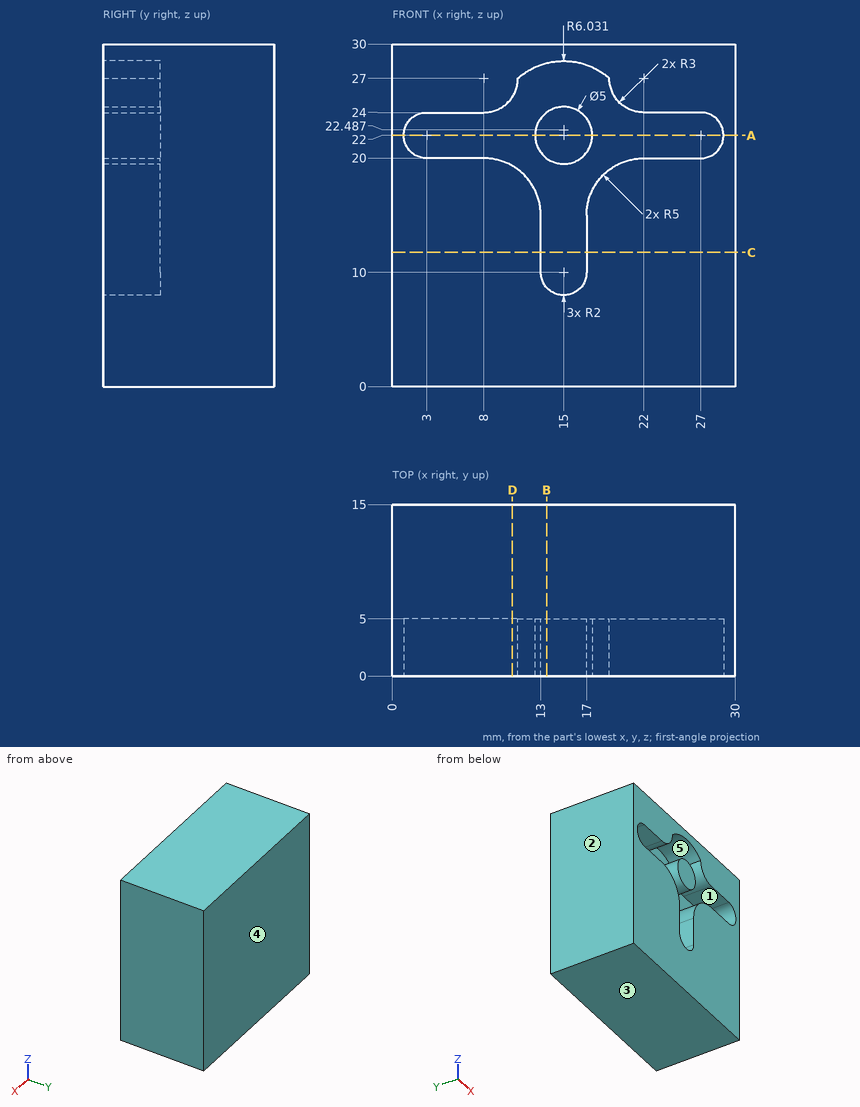
Here's the drawing with two shaded views (mm, measured from the low corner). I have some questions. A direction names the side the tool comes from. Coordinates: 2 decimals unless noted, no trailing zeros. Write each loop counter-clockwise with the first axis right and the second up, starting at its lowest first coordinate (ties: lowest second). Pieces come first, ordered by that corner, then holes.
Item 1: I want a section at C-C on z = 11.75. Write out the boundary of the cut face in (x, y), and give its area (3 significant figures).
Item 2: I want a section at B-B on x = 13.5. Write out the boundary of the cut face in (y, z).
Item 3: If I drill on line 1 (X direction, y = 4.5, z = 14.5); line 2 (Z direction, x = 26.5, y = 0.5); line 3 (Y direction, x = 21.75, z = 23.5), over which ranges is the centre line in solid material (lowest first)?
Item 4: If we mould it in two halves opening along Z, with no side actions, what happens to the marked faces 1, 2 and 3? For each: +Z half, -Z half, draft (parallel to the pull), parting line (faces both ways), or undercut.
Item 5: I want a section at D-D on x = 10.5. Write out the boundary of the cut face in (y, z).
Item 6: On a 3-axis mill with a long thin cutter (end or side, diameter ignored), from which of +Z, -Z, +X, -X, +Y, -Y can I reach the whole of each face in a straight line? I mean the marked faces 4 and 5. Say none if no direction works.
Item 7: I want a section at A-A on z = 22. Write out the boundary of the cut face in (x, y), and give its area (3 significant figures).
Findings below:
1. outline: (0, 0) - (13, 0) - (13, 5) - (17, 5) - (17, 0) - (30, 0) - (30, 15) - (0, 15) - close
1. area: 430 mm2
2. outline: (0, 0) - (15, 0) - (15, 30) - (0, 30) - (0, 28.33) - (5, 28.33) - (5, 24) - (0, 24) - (0, 20) - (5, 20) - (5, 8.68) - (0, 8.68) - close
3. line 1: x = 0 to 13, 17 to 30
3. line 2: z = 0 to 20, 24 to 30
3. line 3: y = 5 to 15
4. face 1: undercut
4. face 2: draft
4. face 3: -Z half
5. outline: (0, 0) - (15, 0) - (15, 30) - (0, 30) - (0, 25.34) - (5, 25.34) - (5, 19.33) - (0, 19.33) - close
6. face 4: +Z, -Z, +X, -X, +Y
6. face 5: -Y
7. outline: (0, 0) - (1, 0) - (1, 5) - (12.5, 5) - (12.5, 0) - (17.5, 0) - (17.5, 5) - (29, 5) - (29, 0) - (30, 0) - (30, 15) - (0, 15) - close
7. area: 335 mm2
